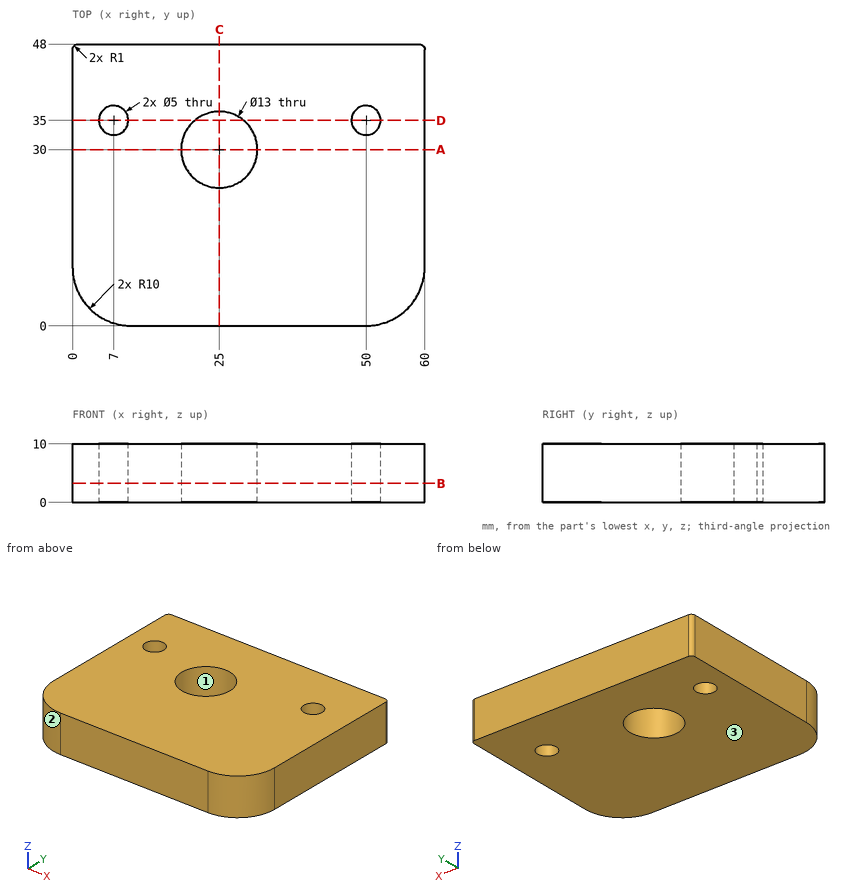
Input: dimensioned drawing with shaded views. Units: mm. Origin: part minimum x, y, z. Round coordinates to 2 decimals unless told otherwise and drop trailing zeros. Order: outer loops, then holes, each group sorted by start corner. A loop starts at its lowest first (then second) coordinate and runs counter-clockwise, first axis right, second up. Notation, with made-up numbers: M 37,-6.75 L 92,-6.75 A17 ccw 92,13.25 Z; hole C 29.5,50.25 d4. An arc over 180 degrees is marked long. Use one line per item in the form item = value. Start each with the question number.
Q1. Material intervals for line 1 (Y direction, x = 25, z = 3.5); line 2 (Y direction, x = 50, z = 1.5); line 3 (X direction, y = 9.5, z = 7.5), sorted ascending. Write a range as [from, to].
Q2. Cut plane D-D (y = 35). Return loops of the section in (x, z).
Q3. Cut plane B-B (z = 3.25). Return loops of the section in (x, y), and give its area (3 significant figures).
Q4. Cut plane A-A (y = 30). Return loops of the section in (x, z).
Q5. Mould query, pull axis X, two halves, no side actions, for the marked faces 1, 2 and 3. Classes: +X half, -X half, draft (parallel to the pull), parting line (faces both ways), or undercut.
Q6. Cut plane C-C (x = 25). Return loops of the section in (y, z).
Geometry results:
q1.line_1 = [0, 23.5], [36.5, 48]
q1.line_2 = [0, 32.5], [37.5, 48]
q1.line_3 = [0.01, 59.99]
q2.outline = M 0,0 L 4.5,0 L 4.5,10 L 0,10 Z; M 9.5,0 L 20.85,0 L 20.85,10 L 9.5,10 Z; M 29.15,0 L 47.5,0 L 47.5,10 L 29.15,10 Z; M 52.5,0 L 60,0 L 60,10 L 52.5,10 Z
q3.outline = M 0,10 A10 ccw 10,0 L 50,0 A10 ccw 60,10 L 60,47 A1 ccw 59,48 L 1,48 A1 ccw 0,47 Z; hole C 7,35 d5; hole C 25,30 d13; hole C 50,35 d5
q3.area = 2,660 mm^2
q4.outline = M 0,0 L 18.5,0 L 18.5,10 L 0,10 Z; M 31.5,0 L 60,0 L 60,10 L 31.5,10 Z
q5.face_1 = undercut
q5.face_2 = -X half
q5.face_3 = draft
q6.outline = M 0,0 L 23.5,0 L 23.5,10 L 0,10 Z; M 36.5,0 L 48,0 L 48,10 L 36.5,10 Z
